For this review, take the finished solid that the model builds, in its own axes (mm). A direction names the side the tool comes from. Coordinates: 2 decimals unless noted, no trailing zeros. Order: outer loops, then holes, each group sorted by start corner. A loop starts at its lowest first (then second) coordinate and runs counter-clockwise, first axis right, second up. Notation, with made-up numbers: (-36.5, 82) - (-32.5, 82) arc R7 cw to (-32.5, 89) - close; hole circle Ø10 at (17.5, 24.5). An arc over 180 degrees is marked (long way). One line per item, written item: value. Start each with the question number.
(1) Mouldability with a two-part tool opening along X and no side actions: class faces 5 (the flat face through (13, 7, 0)), 6 (the cylindrical face through (-13.11, -6.96, 3.34)) as released by +X, released by -X, zero draft, split by the parting line, or undercut.
(2) For faces 1 (the flat face through (8.11, 11.96, 1.21)), 2 (the cylindrical face through (-2.083, 15.864, 17.05)), 3 (the flat face through (0, 15, 0)), 4 (the flat face through (-3.9, 13.77, 1.18)), list the 3-axis set-ups (+Z, -Z, +X, -X, +Y, -Y) from which the entire face can be reached by the end or side of a thin tool; tool diameter is ignored.
(3) To check wall thickness, follow line 1 along Y through (x, z) = (0, 17.25); line 2 along Y through (x, z) = (0.5, 5); line 3 along Z through (x, y) = (-11, 10.5). State the ranges of each line that lie inside material, in increasing order.
(4) Consider section A-A on z = 14.25. Write out the cut boundary in (x, y), then the cut area to 3 significant figures.
(5) Clearance check with flat-ended pins moving along their axes: pin 1 (12 mm diameter, centred on x = -16, z = 8, fed in from +Y); pin 2 (3 mm diameter, centred on x = -7, z = 6, fed in from -Y); pin 3 (2 mm diameter, centred on y = -8, z = 13.5, fed in from +X). State where each tip first meets the part, or that it passes through.
```python
from build123d import *

# Parameters (mm, degrees)
SKETCH1_R           = 21.79955
BOSS_EXTRUDE1_DEPTH = 20.6502
SKETCH2_R           = 12.7
CUT_EXTRUDE1_DEPTH  = 20.6502
SKETCH3_R           = 16.000000004
CUT_EXTRUDE2_DEPTH  = 7.3025
SKETCH4_OUTSIDE_W   = 58.604
SKETCH4_OUTSIDE_H   = 58.604
CUT_EXTRUDE3_DEPTH  = 4.7752
CUT_EXTRUDE4_DEPTH  = 9.8552
CIRPATTERN1_COUNT   = 17
FILLET1_R           = 0.635


with BuildPart() as part:
    # Sketch1 → Boss-Extrude1 (new body)
    with BuildSketch(Plane.XY):
        Circle(SKETCH1_R)
    extrude(amount=BOSS_EXTRUDE1_DEPTH)

    # Sketch2 → Cut-Extrude1 (cut)
    with BuildSketch(Plane.XY.offset(20.6502)):
        Circle(SKETCH2_R)
    extrude(amount=-CUT_EXTRUDE1_DEPTH, mode=Mode.SUBTRACT)

    # Sketch3 → Cut-Extrude2 (cut)
    with BuildSketch(Plane.XY.offset(20.6502)):
        Circle(SKETCH3_R)
    extrude(amount=-CUT_EXTRUDE2_DEPTH, mode=Mode.SUBTRACT)

    # Sketch4 outside → Cut-Extrude3 (cut)
    with BuildSketch(Plane(origin=(0, 0, 0), x_dir=(-1, 0, 0), z_dir=(0, 0, -1))):
        Rectangle(SKETCH4_OUTSIDE_W, SKETCH4_OUTSIDE_H)
        Polygon((17.661795398, -4.907322758), (13.080763872, 12.841902112), (-4.581031526, 17.74922487), (-17.661795398, 4.907322758), (-13.080763872, -12.841902112), (4.581031526, -17.74922487), align=None, mode=Mode.SUBTRACT)
    extrude(amount=-CUT_EXTRUDE3_DEPTH, mode=Mode.SUBTRACT)

    # Sketch5 → Cut-Extrude4 (cut, symmetric)
    with BuildSketch(Plane(origin=(-15.371279635, 3.967289677, 0), x_dir=(0, 0, 1), z_dir=(-0.9682695833030739, 0.24990801117629627, 0))):
        with BuildLine():
            Line((2.3876, 0.9525), (0, 0.9525))
            Line((0, 0.9525), (0, -0.9525))
            Line((0, -0.9525), (2.3876, -0.9525))
            ThreePointArc((2.3876, -0.9525), (3.3401, 0), (2.3876, 0.9525))
        make_face()
    cut_extrude4 = extrude(amount=CUT_EXTRUDE4_DEPTH, both=True, mode=Mode.SUBTRACT)

    # CirPattern1: Cut-Extrude4 ×17 about axis
    cirpattern1_axis = Axis((0, 0, 0), (0, 0, 1))
    for i in range(1, CIRPATTERN1_COUNT):
        add(cut_extrude4.rotate(cirpattern1_axis, i * 360 / CIRPATTERN1_COUNT), mode=Mode.SUBTRACT)

    # Fillet1
    fillet1_edges = [part.edges().sort_by_distance(p)[0] for p in [
        (-17.661795398, -4.907322758, 2.3876),
        (-13.080763872, 12.841902112, 2.3876),
        (4.581031526, 17.74922487, 2.3876),
        (17.661795398, 4.907322758, 3.964999961),
        (13.080763872, -12.841902112, 3.964999961),
        (-4.581031526, -17.74922487, 2.3876),
    ]]
    fillet(fillet1_edges, radius=FILLET1_R)


solid = part.part
```
Geometry check:
1. face 5: zero draft
1. face 6: undercut
2. face 1: -Z
2. face 2: +Z
2. face 3: -Z, +X, -X, +Y, -Y
2. face 4: -Z, +Y
3. line 1: y = -21.8 to -16, 16 to 21.8
3. line 2: y = -21.79 to -12.69, 12.69 to 21.79
3. line 3: z = 0 to 13.35
4. outline: circle Ø43.6 at (0, 0); hole circle Ø32 at (0, 0)
4. area: 689 mm^2
5. pin 1: stops at y = 19.37
5. pin 2: stops at y = -21.09
5. pin 3: stops at x = 20.65
